from build123d import *

# Parameters (mm, degrees)
SKETCH1_W           = 114.3
SKETCH1_H           = 114.3
SKETCH1_W_2         = 53.975
SKETCH1_H_2         = 9.525
SKETCH1_W_3         = 3.175
SKETCH1_H_3         = 25.4
SKETCH1_H_4         = 25.936362634
BOSS_EXTRUDE1_DEPTH = 3.175


with BuildPart() as part:
    # Sketch1 → Boss-Extrude1 (new body)
    with BuildSketch(Plane(origin=(0, 0, 0), x_dir=(1, 0, 0), z_dir=(0, 1, 0))):
        Rectangle(SKETCH1_W, SKETCH1_H)
        Polygon((-13.1953, -28.132309502), (-13.1953, 0), (13.1953, 0), (13.1953, -28.132309502), (16.3703, -28.132309502), (16.3703, 3.175), (-16.3703, 3.175), (-16.3703, -28.132309502), align=None, mode=Mode.SUBTRACT)
        with Locations((-17.4625, 39.6875)):
            Rectangle(SKETCH1_W_2, SKETCH1_H_2, mode=Mode.SUBTRACT)
        with Locations((-50.8, 39.6875)):
            Rectangle(SKETCH1_W_3, SKETCH1_H_3, mode=Mode.SUBTRACT)
        with Locations((15.875, 39.955681317)):
            Rectangle(SKETCH1_W_3, SKETCH1_H_4, mode=Mode.SUBTRACT)
    extrude(amount=-BOSS_EXTRUDE1_DEPTH)


solid = part.part
Geometry: final body of the model. Coordinates: model frame, mm. A direction names the side the tool comes from. Give positions to 0.01 mm unless a question says otherwise; leave off trailing zeros. Write each loop counter-clockwise with the first axis right and the second up, starting at its lowest first coordinate (ties: lowest second). Pieces come first, ordered by that corner, then holes. Notation, with made-up numbers: (79, 53) -> (107, 53) arc R24 cw to (107, 89) -> close; hole circle Ø6 at (48.25, 54.25). An arc over 180 degrees is marked (long way). Answer in a Markdown table with one row per item.
(1) Set-up query: faces 1 (the flat face through (-44.45, -2, -40)), 2 (the flat face through (-1, -3.175, 12)). Return all of +Z, -Z, +X, -X, +Y, -Y with unobstructed straight access to the full face (end or side cutting, diameter ignored); none if empty.
Answers below:
| item | result |
|---|---|
| face 1 | +Y, -Y |
| face 2 | +Z, -Z, +X, -X, -Y |
(2) Section query D-D on x = -8.5. Return loops of the section in (y, z) (3 decimals), then the cut area to 3 significant figures.
Answers below:
| item | result |
|---|---|
| outline | (-3.175, -57.15) -> (0, -57.15) -> (0, -44.45) -> (-3.175, -44.45) -> close; (-3.175, -34.925) -> (0, -34.925) -> (0, -3.175) -> (-3.175, -3.175) -> close; (-3.175, 0) -> (0, 0) -> (0, 57.15) -> (-3.175, 57.15) -> close |
| area | 323 mm^2 |
(3) Draft query along Z for faces 3 (the flat face through (9.525, -2, -40)), 4 (the flat face through (-1, -2, 57.15)), 5 (the flat face through (15, -2, 28.132)), 6 (the flat face through (57.15, -2, 1)). Return one class per face: +Z half, -Z half, draft (parallel to the pull), parting line (faces both ways), or undercut.
Answers below:
| item | result |
|---|---|
| face 3 | undercut |
| face 4 | +Z half |
| face 5 | undercut |
| face 6 | draft |
(4) Section query B-B on x = -31.5. Return loops of the section in (y, z) (3 decimals), then the cut area to 3 significant figures.
Answers below:
| item | result |
|---|---|
| outline | (-3.175, -57.15) -> (0, -57.15) -> (0, -44.45) -> (-3.175, -44.45) -> close; (-3.175, -34.925) -> (0, -34.925) -> (0, 57.15) -> (-3.175, 57.15) -> close |
| area | 333 mm^2 |
(5) Section query A-A on z = 8. Return loops of the section in (x, y) (3 decimals).
Answers below:
| item | result |
|---|---|
| outline | (-57.15, -3.175) -> (-16.37, -3.175) -> (-16.37, 0) -> (-57.15, 0) -> close; (-13.195, -3.175) -> (13.195, -3.175) -> (13.195, 0) -> (-13.195, 0) -> close; (16.37, -3.175) -> (57.15, -3.175) -> (57.15, 0) -> (16.37, 0) -> close |
(6) Ray query, line 1 along X through (y, z) = (-1.85, 17.5); line 2 along Z through (x, y) = (-11.5, -2.85) (3 decimals); line 3 along X through (y, z) = (-3, -34.5). Return the intervals inside material, ascending. Write a range as [from, to].
Answers below:
| item | result |
|---|---|
| line 1 | [-57.15, -16.37], [-13.2, 13.2], [16.37, 57.15] |
| line 2 | [-57.15, -44.45], [-34.925, -3.175], [0, 57.15] |
| line 3 | [-57.15, -52.39], [-49.21, 14.29], [17.46, 57.15] |
(7) Section query C-C on y = -1.8. State how many separate pieces and enclosed holes the cut face has, then the cut area to 3 significant figures.
Answers below:
| item | result |
|---|---|
| separate pieces | 1 |
| enclosed holes | 4 |
| area | 12,100 mm^2 |
